Source: CAD feature listing. Evaluate the final solid. Frame: model axes, mm. A direction names the side the tool comes from. Round coordinates to 2 decimals unless told otherwise and drop trailing zeros. Loops run counter-clockwise (first coordinate to the right, second up) from the corner with the lowest first, then second, coordinate; pieces in that order, holes last. Notation, with made-up numbers: M 25,74 L 53,74 A9 ccw 53,78 Z; hole C 4,41.5 d10. An arc over 180 degrees is marked long. Write each question's results on one line, items separated by ' | '. Start each with the question number.
1. Section B-B on z = 1. Output: boundary loops of the cut face in (x, y), and give its area (3 significant figures).
2. Set-up query: faces 1 (the flat face through (6, 12, 0)), 2 (the flat face through (-9.47, 19, 2.5)). Return all of +Z, -Z, +X, -X, +Y, -Y with unobstructed straight access to the full face (end or side cutting, diameter ignored); none if empty.
3. Section D-D on x = -17. Output: boundary loops of the cut face in (y, z), and give its area (3 significant figures).
4. Section A-A on y = 24. Output: boundary loops of the cut face in (x, z).
5. Ray query, line 1 (X direction, y = 24, z = 1.95); line 2 (X direction, y = 22, z = 2.8); line 3 (X direction, y = 0, z = 3.45). Return the intervals inside material, ascending.
6. Section C-C on y = 15.5. Output: boundary loops of the cut face in (x, z), and give its area (3 significant figures).
7. Contact query for flat-ended pins moving along their axis: pin 1 Ø10 at (x, y) = (-7, 9) entering from -Z; pin 2 Ø1.5 at (y, z) = (-0.5, 3.5) entering from +X; pin 3 Ø6 at (x, y) = (21, 4) entering from -Z; pin 4 Ø1.5 at (x, z) = (20.5, 4.5) entering from -Y. Output: stop coordinate, or through.
8. Draft query along X for faces 3 (the cylindrical face through (-30.348, 32.525, 2.504)), 4 (the flat face through (6, 12, 5.08)), 5 (the cylindrical face through (27.62, 32.43, 2.5)), 6 (the flat face through (19.994, 10.54, 2.504)). Return one class per face: released by +X, released by -X, zero draft, split by the parting line, or undercut.
from build123d import *

# Parameters (mm, degrees)
F4_DEPTH = 5.08


# Not quite as in the source:
# - the program builds the solid bodies; features that only make, move or delete a surface that nothing else refers to are left out


with BuildPart() as f4:
    # F0 (on Top) → F4 (new body)
    with BuildSketch(Plane.XY):
        with BuildLine():
            ThreePointArc((0, 10.0203), (7.0854220795, 7.0854220795), (10.0203, 0))
            Line((10.0203, 0), (30.2514023598, 21.3797036526))
            ThreePointArc((30.2514023598, 21.3797036526), (27.4591098659, 32.5138598171), (16.8107412275, 28.2268356499))
            Line((16.8107412275, 28.2268356499), (0, 10.0203))
        make_face()
        with BuildLine():
            ThreePointArc((-10.0203, 0), (-7.0854220795, 7.0854220795), (0, 10.0203))
            Line((0, 10.0203), (-19.2001006115, 28.2268356499))
            ThreePointArc((-19.2001006115, 28.2268356499), (-30.5143757694, 32.4238900578), (-31.6996835172, 20.4145964235))
            Line((-31.6996835172, 20.4145964235), (-10.0203, 0))
        make_face()
        with BuildLine():
            ThreePointArc((-10.0203, 0), (0, -10.0203), (10.0203, 0))
            ThreePointArc((10.0203, 0), (7.0854220795, 7.0854220795), (0, 10.0203))
            ThreePointArc((0, 10.0203), (-7.0854220795, 7.0854220795), (-10.0203, 0))
        make_face()
    extrude(amount=F4_DEPTH)


solid = f4.part
Taken from the geometry:
1) outline: M -31.7,20.41 L -10.02,0 A10.02 ccw 10.02,0 L 30.25,21.38 A7.61 ccw long 16.81,28.23 L 0,10.02 L -19.2,28.23 A7.62 ccw long Z | area: 1,270 mm^2
2) face 1: -Z, +X, -X, +Y, -Y | face 2: +Z, -Z, +Y
3) outline: M 6.57,0 L 26.14,0 L 26.14,5.08 L 6.57,5.08 Z | area: 99.4 mm^2
4) outline: M -33.84,0 L -14.74,0 L -14.74,5.08 L -33.84,5.08 Z; M 12.91,0 L 31.42,0 L 31.42,5.08 L 12.91,5.08 Z
5) line 1: -33.84 to -14.74, 12.91 to 31.42 | line 2: -32.98 to -12.63, 11.06 to 30.64 | line 3: -10.02 to 10.02
6) outline: M -26.48,0 L -5.78,0 L -5.78,5.08 L -26.48,5.08 Z; M 5.06,0 L 24.69,0 L 24.69,5.08 L 5.06,5.08 Z | area: 205 mm^2
7) pin 1: z = 0 | pin 2: x = 10.26 | pin 3: through | pin 4: y = 10.28
8) face 3: undercut | face 4: zero draft | face 5: undercut | face 6: released by +X
